```python
from build123d import *

# Parameters (mm, degrees)
F1_DEPTH = 692.15
F2_W     = 203.2
F2_H     = 152.4
F3_DEPTH = 6.35
F4_DEPTH = 3.175


with BuildPart() as f1:
    # F0 (on Top) → F1 (new body)
    with BuildSketch(Plane.XY):
        Polygon((38.1, 19.05), (0, 25.4), (-38.1, 19.05), (-38.1, -19.05), (0, -25.4), (38.1, -19.05), align=None)
    extrude(amount=F1_DEPTH)

    # F2 (on face) → F3 (join)
    with BuildSketch(Plane.XY.offset(692.15)):
        Rectangle(F2_W, F2_H)
        Polygon((38.1, 19.05), (38.1, -19.05), (0, -25.4), (-38.1, -19.05), (-38.1, 19.05), (0, 25.4), align=None, mode=Mode.SUBTRACT)
        Polygon((0, -25.4), (38.1, -19.05), (38.1, 19.05), (0, 25.4), (-38.1, 19.05), (-38.1, -19.05), align=None)
    extrude(amount=F3_DEPTH)

    # F4 (cut): a face of the model
    f4_faces = [f1.faces().sort_by_distance(p)[0] for p in [
        (0, 0, 0),
    ]]
    extrude(f4_faces, amount=-F4_DEPTH, mode=Mode.SUBTRACT)


solid = f1.part
```
Build history of the part. All positions in model axes, mm. A direction names the side the tool comes from. Give positions to 0.01 mm unless a question says otherwise; leave off trailing zeros. Loops run counter-clockwise (first coordinate to the right, second up) from the corner with the lowest first, then second, coordinate; pieces in that order, holes last. Notation, with made-up numbers: (-31, 41) -> (-5, 41) arc R22 ccw to (-5, 70) -> close; hole circle Ø2 at (39.25, -11). An arc over 180 degrees is marked (long way). One line per question, with ' | ' between items. Start each with the question number.
1) Probe L1, parallel to Z at x = 42, y = -61.5; L2, parallel to X at y = 17, z = 219.5; L3, parallel to Y at x = -13, z = 484.5. List the from-to ranges inside material, lowest first.
2) Cut at C-C (y = -1.5). Give the cut face in (x, z) (3 decimals).
3) Cut at A-A (x = -9). Give the cut face in (y, z) (3 decimals), plus the area to 3 significant figures.
4) Cut at D-D (y = -43.5). Give the cut face in (x, z), plus the area to 3 significant figures.
5) 3-axis set-ups, long thin cutter, end or side, ignore diameter. For faces 1 (the flat face through (19.32, 22.18, 342.84)), 2 (the flat face through (-18.78, 22.27, 342.84)), 3 (the flat face through (38.1, 0, 343)), 4 (the flat face through (-38.1, 0, 343)), 5 (the flat face through (18.78, -22.27, 342.84)): which of +Z, -Z, +X, -X, +Y, -Y reach the whole face in a straight line?
6) Pin check, flat tips, straight feed: pin 1 (1 mm diameter, centred on y = -5.5, z = 137, fed in from +X); pin 2 (1.5 mm diameter, centred on y = -27, z = 108, fed in from -X); pin 3 (1 mm diameter, centred on x = 74, y = 1.5, fed in from -Z); pin 4 (6 mm diameter, centred on y = -9.5, z = 89, fed in from -X). Stop position of each tip, or through.
7) Cut at B-B (z = 71.5). Give the cut face in (x, y), plus the area to 3 significant figures.
Return value:
1) L1: 692.15 to 698.5 | L2: -38.1 to 38.1 | L3: -23.23 to 23.23
2) outline: (-101.6, 692.15) -> (-38.1, 692.15) -> (-38.1, 3.175) -> (38.1, 3.175) -> (38.1, 692.15) -> (101.6, 692.15) -> (101.6, 698.5) -> (-101.6, 698.5) -> close
3) outline: (-76.2, 692.15) -> (-23.9, 692.15) -> (-23.9, 3.175) -> (23.9, 3.175) -> (23.9, 692.15) -> (76.2, 692.15) -> (76.2, 698.5) -> (-76.2, 698.5) -> close | area: 33,900 mm^2
4) outline: (-101.6, 692.15) -> (101.6, 692.15) -> (101.6, 698.5) -> (-101.6, 698.5) -> close | area: 1,290 mm^2
5) face 1: -Z, +X, +Y | face 2: -Z, -X, +Y | face 3: -Z, +X, +Y, -Y | face 4: -Z, -X, +Y, -Y | face 5: -Z, +X, -Y
6) pin 1: x = 38.1 | pin 2: through | pin 3: z = 692.15 | pin 4: x = -38.1
7) outline: (-38.1, -19.05) -> (0, -25.4) -> (38.1, -19.05) -> (38.1, 19.05) -> (0, 25.4) -> (-38.1, 19.05) -> close | area: 3,390 mm^2
